Read the model definition and answer for the solid it produces. Units are mm, in the model's axes. Face numbers are marked on the shaded views. A direction names the side the tool comes from. Coordinates: 2 decimals unless noted, no trailing zeros. Write each loop counter-clockwise with the first axis right and the second up, starting at its lowest first coordinate (ties: lowest second). Pieces come first, ordered by that corner, then holes. Notation, with made-up numbers: M 0.5,-7 L 4.5,-7 A16 ccw 4.5,10 Z; hole C 69,86.5 d2. An arc over 180 degrees is marked long. Use a Markdown table: item, result. Add a question column.
from build123d import *

# Parameters (mm, degrees)
BOSS_EXTRUDE1_DEPTH = 23.3
BOSS_EXTRUDE2_REACH = 41.551
SKETCH2_W           = 9.3
SKETCH2_H           = 1.6
CUT_EXTRUDE2_DEPTH  = 1.6


with BuildPart() as part:
    # Sketch1 → Boss-Extrude1 (new body)
    with BuildSketch(Plane(origin=(0, 0, 0), x_dir=(0, 0, -1), z_dir=(1, 0, 0))):
        with BuildLine():
            Line((-43.625137797, -16.697262805), (-43.625137797, -15.697262805))
            Line((-43.625137797, -15.697262805), (-16.525137797, -15.697262805))
            Line((-16.525137797, -15.697262805), (-16.525137797, -16.697262805))
            Line((-16.525137797, -16.697262805), (-15.325137797, -16.697262805))
            Line((-15.325137797, -16.697262805), (-15.325137797, -14.097262805))
            Line((-15.325137797, -14.097262805), (-17.575137797, -14.097262805))
            Line((-17.575137797, -14.097262805), (-17.575137797, -12.497262805))
            ThreePointArc((-17.575137797, -12.497262805), (-30.075137797, -13.985375722), (-42.575137797, -12.497262805))
            Line((-42.575137797, -12.497262805), (-42.575137797, -14.097262805))
            Line((-42.575137797, -14.097262805), (-44.825137797, -14.097262805))
            Line((-44.825137797, -14.097262805), (-44.825137797, -16.697262805))
            Line((-44.825137797, -16.697262805), (-43.625137797, -16.697262805))
        make_face()
    extrude(amount=BOSS_EXTRUDE1_DEPTH)

    # Sketch2 → Boss-Extrude2 (add, up to next)
    with BuildSketch(Plane.XY.offset(42.575137797), mode=Mode.PRIVATE) as boss_extrude2_sk1:
        with Locations((11.65, -13.297262805)):
            Rectangle(SKETCH2_W, SKETCH2_H)
    boss_extrude2_tool1 = extrude(boss_extrude2_sk1.sketch, amount=-BOSS_EXTRUDE2_REACH, mode=Mode.PRIVATE) - part.part
    add(boss_extrude2_tool1.solids().sort_by_distance((11.65, -13.297263, 42.575138))[0])

    # Sketch3 → Cut-Extrude2 (cut)
    with BuildSketch(Plane.XZ.offset(15.697262805)):
        with BuildLine():
            ThreePointArc((21.3, 39.625137797), (19.885786438, 40.210924235), (19.3, 41.625137797))
            Line((19.3, 41.625137797), (4, 41.625137797))
            ThreePointArc((4, 41.625137797), (3.414213562, 40.210924235), (2, 39.625137797))
            Line((2, 39.625137797), (2, 38.425137797))
            Line((2, 38.425137797), (9, 38.425137797))
            Line((9, 38.425137797), (9, 21.725137797))
            Line((9, 21.725137797), (2, 21.725137797))
            Line((2, 21.725137797), (2, 20.525137797))
            ThreePointArc((2, 20.525137797), (3.414213562, 19.939351359), (4, 18.525137797))
            Line((4, 18.525137797), (19.3, 18.525137797))
            ThreePointArc((19.3, 18.525137797), (19.885786438, 19.939351359), (21.3, 20.525137797))
            Line((21.3, 20.525137797), (21.3, 21.725137797))
            Line((21.3, 21.725137797), (14.3, 21.725137797))
            Line((14.3, 21.725137797), (14.3, 38.425137797))
            Line((14.3, 38.425137797), (21.3, 38.425137797))
            Line((21.3, 38.425137797), (21.3, 39.625137797))
        make_face()
    extrude(amount=-CUT_EXTRUDE2_DEPTH, mode=Mode.SUBTRACT)


solid = part.part
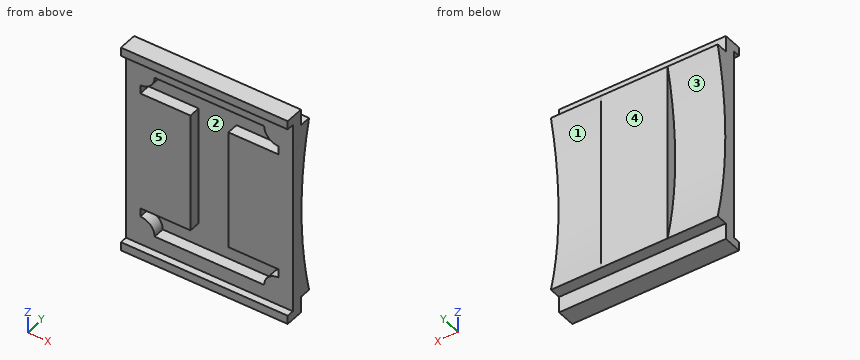
Item 1: For the marked faces 3, 4 and 5, determine the directions among +Z, -Z, +X, -X, +Y, -Y from which every point of the face is accessible in a straight line to the end or side of a thin tool.
Item 2: Determine the mould class of the marked faces 1 and 2 for opening direction X: pulls with the +X half, pulls with the -X half, needs draft (parallel to the pull), parting line crosses it, or undercut.
Item 3: Find section B-B on y = -14.9. Give the vertices of the cut face in (x, z).
Item 4: Each of these flat-tipped pins is pushed along its axis until it touches: pin 1 (1.8 mm diameter, centred on x = 12, z = 44, fed in from +Y); pin 2 (0.5 mm diameter, centred on x = 8.5, y = -13, fed in from -Z); pin 3 (0.8 mm diameter, centred on x = 6, y = -13, fed in from +Z). Where does it stop, or does it pass through?
Item 5: Find section D-D on z = 22.75. Give the vertices of the cut face in (x, y).
Item 6: Find section A-A on y = -16.25. Give the vertices of the cut face in (x, z), then the cut area to 3 significant figures.
Item 7: Consider probe 1 along Z at (x, y) = (14.5, -14.7); probe 2 along Z at (x, y) = (20.75, -16.5); probe 3 along X at (y, z) = (-15, 32.75). Determine where each line is inside the solid, lowest interval first.
Item 8: Find section C-C on x = 8.5. Give the vertices of the cut face in (y, z).
Geometry says:
| question | item | result |
|---|---|---|
| 1 | face 3 | -X, +Y |
| 1 | face 4 | +Z, -Z, +X, -X, +Y |
| 1 | face 5 | +X, -X, -Y |
| 2 | face 1 | needs draft |
| 2 | face 2 | undercut |
| 3 | outline | M 0,15.33 L 23.3,15.33 L 23.3,44.83 L 0,44.83 Z; hole M 2,20.53 A2 cw 4,18.53 L 19.3,18.53 A2 cw 21.3,20.53 L 21.3,21.73 L 14.3,21.73 L 14.3,38.43 L 21.3,38.43 L 21.3,39.63 A2 cw 19.3,41.63 L 4,41.63 A2 cw 2,39.63 L 2,38.43 L 9,38.43 L 9,21.73 L 2,21.73 Z |
| 4 | pin 1 | stops at y = -14.1 |
| 4 | pin 2 | stops at z = 17.58 |
| 4 | pin 3 | stops at z = 42.58 |
| 5 | outline | M 0,-15.7 L 9,-15.7 L 9,-14.1 L 14.3,-14.1 L 14.3,-15.7 L 23.3,-15.7 L 23.3,-13.48 L 16.3,-13.48 L 16.3,-12.5 L 7,-12.5 L 7,-13.48 L 0,-13.48 Z |
| 6 | outline | M 0,15.33 L 23.3,15.33 L 23.3,16.53 L 0,16.53 Z; M 0,43.63 L 23.3,43.63 L 23.3,44.83 L 0,44.83 Z |
| 6 | area | 55.9 mm2 |
| 7 | probe 1 | z = 15.33 to 18.53, 21.73 to 38.43, 41.63 to 44.83 |
| 7 | probe 2 | z = 15.33 to 16.53, 43.63 to 44.83 |
| 7 | probe 3 | x = 0 to 9, 14.3 to 23.3 |
| 8 | outline | M -16.7,15.33 L -14.1,15.33 L -14.1,17.58 L -12.5,17.58 L -12.5,42.58 L -14.1,42.58 L -14.1,44.83 L -16.7,44.83 L -16.7,43.63 L -15.7,43.63 L -15.7,41.63 L -14.1,41.63 L -14.1,38.43 L -15.7,38.43 L -15.7,21.73 L -14.1,21.73 L -14.1,18.53 L -15.7,18.53 L -15.7,16.53 L -16.7,16.53 Z |
